The model under review builds one solid part; all positions refer to its coordinate system, in mm. Round coordinates to 2 decimals unless told otherwise and drop trailing zeros. Order: outer loops, then holes, each group sorted by start corner. A loop starts at its lowest first (then second) coordinate and runs counter-clockwise, first axis right, second up. Notation, with made-up numbers: M 74.25,-2.5 L 108.25,-2.5 A23 ccw 108.25,26.5 Z; hole C 4.5,47.5 d4. An arc over 180 degrees is marked long. Use a Markdown table: item, result. Add a question column.
1. To check wall thickness, follow probe 1 along Y at (x, z) = (4, 0); probe 2 along Z at (x, y) = (3.5, -23); probe 3 along Z at (x, y) = (6.5, -8). State the ranges of each line that lie inside material, in increasing order.
2. Consider section B-B on x = 1.25. Count the separate pieces of the cut face and the enclosed holes in it, then the cut area to 3 significant figures.
3. Consider section A-A on y = 0. State the section outline as (x, z) points.
4. Insertion check: P1, Ø2.5, axis at y = 0, z = 8, coming from the -X side; P2, Ø4, axis at x = 4, y = -15.5, coming from the +Z side; P3, Ø1, axis at x = 6.5, z = 10.5, coming from the +Y side. Each pin has a flat end and moves straight along its axis. Give the tip position at first contact, or say it passes through.
5. Consider section C-C on z = -23. State the section outline as (x, y) points.
6. Consider section D-D on z = -8. State the section outline as (x, y) points, then the cut area to 3 significant figures.
from build123d import *

# Parameters (mm, degrees)
SPROCKET_R                   = 45.5
ESTRUSIONE_ESTRUSIONE2_DEPTH = 8
SCHIZZO1_R                   = 5
SCHIZZO1_R_2                 = 1.5
TAGLIO_ESTRUSIONE2_DEPTH     = 9


with BuildPart() as part:
    # Sprocket → Estrusione-Estrusione2 (new body)
    with BuildSketch(Plane(origin=(0, 0, 0), x_dir=(0, 0, -1), z_dir=(1, 0, 0))):
        Circle(SPROCKET_R)
    extrude(amount=ESTRUSIONE_ESTRUSIONE2_DEPTH)

    # Schizzo1 → Taglio-Estrusione2 (cut, through all)
    with BuildSketch(Plane(origin=(0, 0, 0), x_dir=(0, 0, -1), z_dir=(1, 0, 0))):
        Circle(SCHIZZO1_R)
        with Locations((0, 23)):
            Circle(SCHIZZO1_R_2)
        with Locations((8, 0)):
            Circle(SCHIZZO1_R_2)
        with Locations((0, 8)):
            Circle(SCHIZZO1_R_2)
        with Locations((23, 0)):
            Circle(SCHIZZO1_R_2)
        with Locations((0, -8)):
            Circle(SCHIZZO1_R_2)
        with Locations((0, -23)):
            Circle(SCHIZZO1_R_2)
        with Locations((-8, 0)):
            Circle(SCHIZZO1_R_2)
        with Locations((-23, 0)):
            Circle(SCHIZZO1_R_2)
    extrude(amount=TAGLIO_ESTRUSIONE2_DEPTH, mode=Mode.SUBTRACT)


solid = part.part
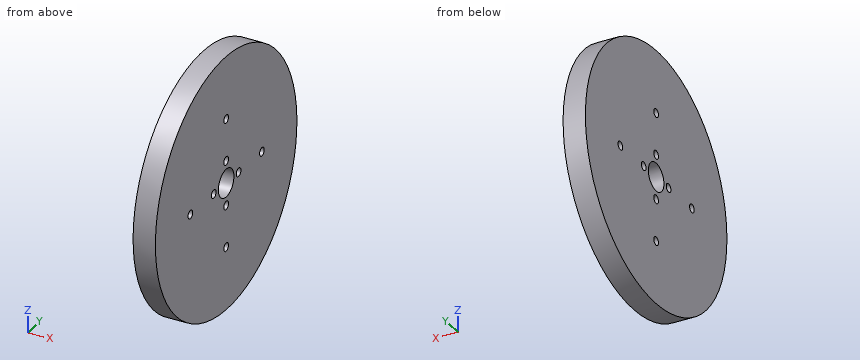
Answer block:
| question | item | result |
|---|---|---|
| 1 | probe 1 | -45.5 to -24.5, -21.5 to -9.5, -6.5 to -5, 5 to 6.5, 9.5 to 21.5, 24.5 to 45.5 |
| 1 | probe 2 | -39.26 to -1.5, 1.5 to 39.26 |
| 1 | probe 3 | -44.79 to -1.5, 1.5 to 44.79 |
| 2 | separate pieces | 1 |
| 2 | enclosed holes | 9 |
| 2 | area | 6,370 mm^2 |
| 3 | outline | M 0,-45.5 L 8,-45.5 L 8,-24.5 L 0,-24.5 Z; M 0,-21.5 L 8,-21.5 L 8,-9.5 L 0,-9.5 Z; M 0,-6.5 L 8,-6.5 L 8,-5 L 0,-5 Z; M 0,5 L 8,5 L 8,6.5 L 0,6.5 Z; M 0,9.5 L 8,9.5 L 8,21.5 L 0,21.5 Z; M 0,24.5 L 8,24.5 L 8,45.5 L 0,45.5 Z |
| 4 | P1 | through |
| 4 | P2 | z = 43.45 |
| 4 | P3 | y = 44.39 |
| 5 | outline | M 0,-39.26 L 8,-39.26 L 8,-1.5 L 0,-1.5 Z; M 0,1.5 L 8,1.5 L 8,39.26 L 0,39.26 Z |
| 6 | outline | M 0,-44.79 L 8,-44.79 L 8,-1.5 L 0,-1.5 Z; M 0,1.5 L 8,1.5 L 8,44.79 L 0,44.79 Z |
| 6 | area | 693 mm^2 |
